Read the model definition and answer for the solid it produces. Units are mm, in the model's axes. A direction names the side the tool comes from. Give positions to 0.01 mm unless a question says otherwise; leave off trailing zeros. Order: outer loops, then holes, each group sorted by start corner. A loop starts at its lowest first (then second) coordinate and runs counter-clockwise, first axis right, second up.
```python
from build123d import *

# Parameters (mm, degrees)
F0_W     = 406.4
F0_H     = 330.2
F1_DEPTH = 165.1
F3_DEPTH = 406.401
F4_T     = -19.05


with BuildPart() as f1:
    # F0 (on Front) → F1 (new body, symmetric)
    with BuildSketch(Plane.XZ):
        Rectangle(F0_W, F0_H)
    extrude(amount=F1_DEPTH, both=True)

    # F2 (on face) → F3 (cut, through all)
    with BuildSketch(Plane.YZ.offset(203.2)):
        Polygon((165.1, 165.1), (-165.1, 165.1), (-165.1, 88.9), align=None)
    extrude(amount=-F3_DEPTH, mode=Mode.SUBTRACT)

    # F4
    f4_openings = [f1.faces().sort_by_distance(p)[0] for p in [
        (0, 0, 127),
    ]]
    offset(amount=F4_T, openings=f4_openings)


solid = f1.part
```
1) Consider L1, parallel to X at y = -71, z = 64.5; L2, parallel to Y at x = 99.5, z = 7.5. Determine where each line is inside the solid, lowest interval first.
Final values:
L1: x = -203.2 to -184.15, 184.15 to 203.2
L2: y = -165.1 to -146.05, 146.05 to 165.1
2) Given pin 1 (1.5 mm diameter, centred on x = 130, z = 125, fed in from -Y), flat-ended and moving along its own axis, determine where the tip first touches the part or whether it passes through.
Final values:
pin 1: stops at y = 146.05
3) A tool of negligible diameter and unlimited length cuts with its end or side. For faces 4 (the face through (-184.15, -2, 5)), 5 (the face through (-3, -165.1, -36)), from which of +Z, -Z, +X, -X, +Y, -Y can it reach the whole face along a straight path? Write none if from no direction.
Final values:
face 4: +Z
face 5: +Z, -Z, +X, -X, -Y
4) For a pull along X with two mould halves and no side action, classify faces 1 (the face through (-3, 165.1, 2)), 2 (the face through (-3, 146.05, 9)), 3 (the face through (203.2, -2, -2)) as released by +X, released by -X, zero draft, split by the parting line, or undercut.
Final values:
face 1: zero draft
face 2: undercut
face 3: released by +X
5) The part is cut by section B-B on x = -26.5. Determine the outline of the cut face in (y, z).
Final values:
outline: (-165.1, -165.1) - (165.1, -165.1) - (165.1, 165.1) - (146.05, 160.7) - (146.05, -146.05) - (-146.05, -146.05) - (-146.05, 93.3) - (-165.1, 88.9) - close
6) The part is cut by section A-A on z = -132.5. Determine the outline of the cut face in (x, y), and give its area (3 significant figures).
Final values:
outline: (-203.2, -165.1) - (203.2, -165.1) - (203.2, 165.1) - (-203.2, 165.1) - close; hole (-184.15, -146.05) - (184.15, -146.05) - (184.15, 146.05) - (-184.15, 146.05) - close
area: 26,600 mm2
7) The part is cut by section C-C on y = 45.5. Determine the outline of the cut face in (x, z), and give its area (3 significant figures).
Final values:
outline: (-203.2, -165.1) - (203.2, -165.1) - (203.2, 137.5) - (184.15, 137.5) - (184.15, -146.05) - (-184.15, -146.05) - (-184.15, 137.5) - (-203.2, 137.5) - close
area: 18,500 mm2
